Input: part model. Units: mm. Frame: model coordinates. A direction names the side the tool comes from. Coordinates: 2 decimals unless noted, no trailing zeros. Loops run counter-clockwise (first coordinate to the right, second up) from the corner with the lowest first, then second, coordinate; pieces in that order, holes last.
Item 1: Section B-B on y = -5.5. Return loops of the section in (x, z), and give its area (3 significant figures).
Item 2: Reachability of faces 1 (the cylindrical face through (54.315, -1.346, -5.626)), 2 (the cylindrical face through (0.87, -1.35, -5.65)), 3 (the flat face through (27, 0, -2)), 4 (the flat face through (28, -1, -6)) from +Z, -Z, +X, -X, +Y, -Y: full face, straight path, thin tool, end or side. Return the list, or none.
Item 3: Section D-D on z = -7.5. Return loops of the section in (x, y), and give its area (3 significant figures).
Item 4: Contact query for flat-ended pins moving along their axis: P1, Ø3, axis at x = 49.5, z = -7, coming from the +Y side; P2, Ø2.5, axis at x = 21.5, z = -3, coming from the -Y side; P3, Ø2.5, axis at x = 14, z = -8, coming from the +Y side; P4, Ø4, axis at y = -2, z = -5.5, coming from the +X side. Output: stop coordinate, or through.
Item 5: Section A-A on x = 28. Return loops of the section in (y, z).
Item 6: Ray query, line 1 along Y through (x, z) = (17, -1.5); line 2 along Y through (x, z) = (18, -6.25); line 3 along Z through (x, y) = (44, -2.5). Return the intervals inside material, ascending.
Item 7: Section C-C on z = -1.25. Return loops of the section in (x, y).
```python
from build123d import *

# Parameters (mm, degrees)
BOSS_EXTRUDE1_DEPTH = 2
BOSS_EXTRUDE2_START = -8.6
BOSS_EXTRUDE2_DEPTH = 8.6
BOSS_EXTRUDE3_DEPTH = 2
SKETCH8_W           = 55.15
SKETCH8_H           = 4.9
CUT_EXTRUDE3_DEPTH  = 57.436535152


with BuildPart() as part:
    # Sketch1 → Boss-Extrude1 (new body)
    with BuildSketch(Plane(origin=(0, 0, 0), x_dir=(1, 0, 0), z_dir=(0, 1, 0))):
        with BuildLine():
            Line((2, 0), (53.15, 0))
            ThreePointArc((53.15, 0), (54.564213562, 0.585786438), (55.15, 2))
            Line((55.15, 2), (55.15, 4))
            ThreePointArc((55.15, 4), (54.564213562, 5.414213562), (53.15, 6))
            Line((53.15, 6), (2, 6))
            ThreePointArc((2, 6), (0.585786438, 5.414213562), (0, 4))
            Line((0, 4), (0, 2))
            ThreePointArc((0, 2), (0.585786438, 0.585786438), (2, 0))
        make_face()
    extrude(amount=BOSS_EXTRUDE1_DEPTH)

    # Sketch2 → Boss-Extrude2 (add)
    with BuildSketch(Plane(origin=(0, 2, 0), x_dir=(1, 0, 0), z_dir=(0, 1, 0)).offset(BOSS_EXTRUDE2_START)):
        with BuildLine():
            Line((1.6, 0.040408206), (1.6, 2.5))
            ThreePointArc((1.6, 2.5), (2.302943725, 4.197056275), (4, 4.9))
            Line((4, 4.9), (51.15, 4.9))
            ThreePointArc((51.15, 4.9), (52.847056275, 4.197056275), (53.55, 2.5))
            Line((53.55, 2.5), (53.55, 0.040408206))
            ThreePointArc((53.55, 0.040408206), (54.699193338, 0.735088936), (55.15, 2))
            Line((55.15, 2), (55.15, 4))
            ThreePointArc((55.15, 4), (54.564213562, 5.414213562), (53.15, 6))
            Line((53.15, 6), (2, 6))
            ThreePointArc((2, 6), (0.585786438, 5.414213562), (0, 4))
            Line((0, 4), (0, 2))
            ThreePointArc((0, 2), (0.450806662, 0.735088936), (1.6, 0.040408206))
        make_face()
    extrude(amount=BOSS_EXTRUDE2_DEPTH)

    # Sketch4 → Boss-Extrude3 (add)
    with BuildSketch(Plane.XZ.offset(6.6)):
        with BuildLine():
            Line((0, -4), (0, -8))
            ThreePointArc((0, -8), (0.585786438, -9.414213562), (2, -10))
            Line((2, -10), (53.15, -10))
            ThreePointArc((53.15, -10), (54.564213562, -9.414213562), (55.15, -8))
            Line((55.15, -8), (55.15, -4))
            ThreePointArc((55.15, -4), (54.564213562, -5.414213562), (53.15, -6))
            Line((53.15, -6), (2, -6))
            ThreePointArc((2, -6), (0.585786438, -5.414213562), (0, -4))
        make_face()
    extrude(amount=-BOSS_EXTRUDE3_DEPTH)

    # Sketch8 → Cut-Extrude3 (cut, through all)
    with BuildSketch(Plane.XZ):
        with Locations((27.575, -2.45)):
            Rectangle(SKETCH8_W, SKETCH8_H)
    extrude(amount=CUT_EXTRUDE3_DEPTH, mode=Mode.SUBTRACT)


solid = part.part
```
Results found:
1. outline: (0, -8) arc R2 ccw to (2, -10) - (53.15, -10) arc R2 ccw to (55.15, -8) - (55.15, -4.9) - (0, -4.9) - close
1. area: 280 mm2
2. face 1: -Z, +X, +Y
2. face 2: -Z, -X, +Y
2. face 3: +Z, +X, -X, -Y
2. face 4: -Z, +X, -X, +Y
3. outline: (0, -6.6) - (55.15, -6.6) - (55.15, -4.6) - (0, -4.6) - close
3. area: 110 mm2
4. P1: stops at y = 2
4. P2: stops at y = 0
4. P3: stops at y = -4.6
4. P4: stops at x = 54.94
5. outline: (-6.6, -10) - (-4.6, -10) - (-4.6, -6) - (2, -6) - (2, 0) - (0, 0) - (0, -4.9) - (-6.6, -4.9) - close
6. line 1: y = 0 to 2
6. line 2: y = -6.6 to -4.6
6. line 3: z = -6 to -4.9
7. outline: (0.15, 0) - (55, 0) - (55, 2) - (0.15, 2) - close
